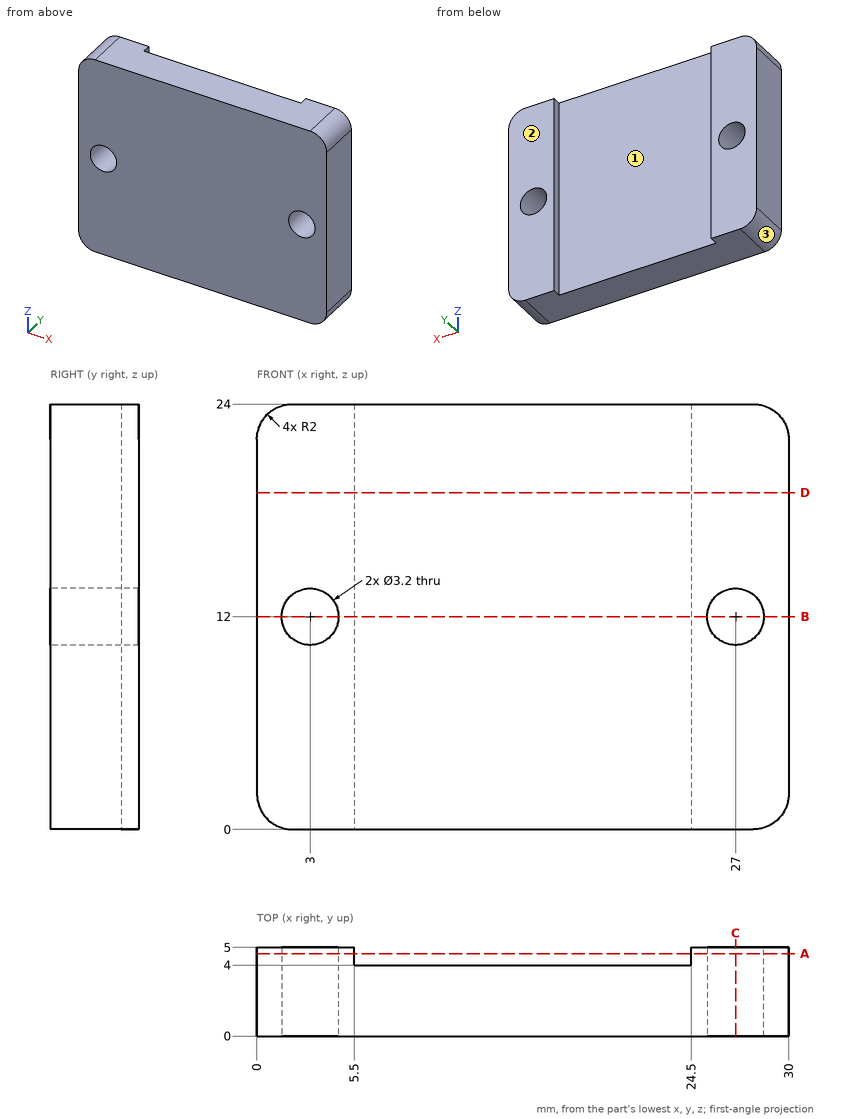
The figure shows three views and two pictorial views of one solid part (mm, origin at its lowest corner). Answer the questions. Round coordinates to 2 decimals unless told otherwise and drop trailing zeros. Order: outer loops, then holes, each group sorted by start corner. A loop starts at its lowest first (then second) coordinate and runs counter-clockwise, first axis right, second up. Notation, with made-up numbers: (42, 7.5) -> (78, 7.5) arc R24 ccw to (78, 39.5) -> close; hole circle Ø6 at (72, 84.25). An arc over 180 degrees is marked (long way). Put each result on its own line as item: value.
Q1. Section C-C, the plane x = 27 is taken. Write down the section's boundary in (y, z), and give its area (3 significant figures).
Results list:
outline: (0, 0) -> (5, 0) -> (5, 10.4) -> (0, 10.4) -> close; (0, 13.6) -> (5, 13.6) -> (5, 24) -> (0, 24) -> close
area: 104 mm^2
Q2. Section B-B, the plane z = 12 is taken. Write down the section's boundary in (x, y).
Results list:
outline: (0, 0) -> (1.4, 0) -> (1.4, 5) -> (0, 5) -> close; (4.6, 0) -> (25.4, 0) -> (25.4, 5) -> (24.5, 5) -> (24.5, 4) -> (5.5, 4) -> (5.5, 5) -> (4.6, 5) -> close; (28.6, 0) -> (30, 0) -> (30, 5) -> (28.6, 5) -> close
Q3. Determine the mould class of the marked faces 1, 2 and 3 for opening direction X: pulls with the +X half, pulls with the -X half, needs draft (parallel to the pull), parting line crosses it, or undercut.
Results list:
face 1: undercut
face 2: needs draft
face 3: pulls with the -X half
Q4. This flat-tipped pin is pushed along its axis until it touches: P1, Ø1, axis at x = 16.5, z = 2.5, coming from the +Y side. Where does it stop, or does it pass through?
Results list:
P1: y = 4
Q5. Consider line 1 along X through (y, z) = (1.5, 12); line 2 along X through (y, z) = (4.4, 9.75); line 3 along Z through (x, y) = (3, 3.1). Determine where each line is inside the solid, lowest interval first.
Results list:
line 1: 0 to 1.4, 4.6 to 25.4, 28.6 to 30
line 2: 0 to 5.5, 24.5 to 30
line 3: 0 to 10.4, 13.6 to 24
Q6. Section A-A, the plane y = 4.65 is taken. Write down the section's boundary in (x, z), and give its area (3 significant figures).
Results list:
outline: (0, 2) arc R2 ccw to (2, 0) -> (5.5, 0) -> (5.5, 24) -> (2, 24) arc R2 ccw to (0, 22) -> close; (24.5, 0) -> (28, 0) arc R2 ccw to (30, 2) -> (30, 22) arc R2 ccw to (28, 24) -> (24.5, 24) -> close; hole circle Ø3.2 at (3, 12); hole circle Ø3.2 at (27, 12)
area: 244 mm^2
Q7. Section D-D, the plane z = 19 is taken. Write down the section's boundary in (x, y).
Results list:
outline: (0, 0) -> (30, 0) -> (30, 5) -> (24.5, 5) -> (24.5, 4) -> (5.5, 4) -> (5.5, 5) -> (0, 5) -> close
